Can you work these out from the model? Positions are in its coordinate system, mm. Coordinates: 2 decimals unless noted, no trailing zeros. Order: outer loops, then holes, each group sorted by start corner. A loop starts at its lowest first (then second) coordinate and runs counter-clockwise, first axis right, second up.
```python
from build123d import *

# Parameters (mm, degrees)
SKETCH_1_W                  = 85
SKETCH_1_H                  = 90
EXTRUDE_1_DEPTH             = 80
SKETCH_2_W                  = 75
SKETCH_2_H                  = 80
CUT_EXTRUDE_1_DEPTH         = 148.39402973
HOLE_WIZARD_6_6_6_6_1_D     = 6.6
HOLE_WIZARD_6_0_6_1_D       = 6
HOLE_WIZARD_6_0_6_1_DEPTH   = 85
HOLE_WIZARD_2_0_2_1_D       = 2
HOLE_WIZARD_4_5_4_5_1_D     = 4.5
HOLE_WIZARD_4_5_4_5_1_DEPTH = 90
HOLE_WIZARD_3_4_3_4_1_D     = 3.4
HOLE_WIZARD_3_4_3_4_1_DEPTH = 90
CHAMFER_1_SIZE              = 3
CHAMFER_2_SIZE              = 2.45
CHAMFER_3_SIZE              = 1.45


with BuildPart() as part:
    # 草圖1 → 填料-伸長1 (new body)
    with BuildSketch(Plane.XZ):
        with Locations((42.5, 45)):
            Rectangle(SKETCH_1_W, SKETCH_1_H)
    extrude(amount=-EXTRUDE_1_DEPTH)

    # 草圖2 → 除料-伸長1 (cut, through all)
    with BuildSketch(Plane(origin=(0, 80, 0), x_dir=(-1, 0, 0), z_dir=(0, 1, 0))):
        with Locations((-47.5, 40)):
            Rectangle(SKETCH_2_W, SKETCH_2_H)
    extrude(amount=-CUT_EXTRUDE_1_DEPTH, mode=Mode.SUBTRACT)

    # Ø6.6 (6.6) 直徑孔1 (through all)
    with Locations(Plane(origin=(10, 0, 0), x_dir=(0, 0, -1), z_dir=(1, 0, 0))):
        with Locations((-38.807552288, 10.023708227), (-60.353251324, 17.960372949), (-69.976291773, 38.807552288), (-62.039627051, 60.353251324), (-41.192447712, 69.976291773), (-19.646748676, 62.039627051), (-10.023708227, 41.192447712), (-17.960372949, 19.646748676)):
            Hole(HOLE_WIZARD_6_6_6_6_1_D / 2)

    # Ø6.0 (6) 直徑孔1
    with Locations(Plane.ZY):
        with Locations((12.761847554, 52.57310826), (67.238152446, 27.42689174)):
            Hole(HOLE_WIZARD_6_0_6_1_D / 2, depth=HOLE_WIZARD_6_0_6_1_DEPTH)

    # Ø2.0 (2) 直徑孔1 (through all)
    with Locations(Plane(origin=(0, 0, 80), x_dir=(-1, 0, 0), z_dir=(0, 0, -1))):
        with Locations((-46.377364171, 55.211997886), (-65.622635829, 24.788002114)):
            Hole(HOLE_WIZARD_2_0_2_1_D / 2)

    # Ø4.5 (4.5) 直徑孔1
    with Locations(Plane.XY.offset(90)):
        with Locations((71.275302439, 31.985785415), (41.421835359, 30.77830733), (55.302862202, 57.235907255)):
            Hole(HOLE_WIZARD_4_5_4_5_1_D / 2, depth=HOLE_WIZARD_4_5_4_5_1_DEPTH)

    # Ø3.4 (3.4) 直徑孔1
    with Locations(Plane.XY.offset(90)):
        with Locations((48.134653009, 24.375137866), (38.51201718, 39.587135752)):
            Hole(HOLE_WIZARD_3_4_3_4_1_D / 2, depth=HOLE_WIZARD_3_4_3_4_1_DEPTH)

    # 導角1
    chamfer_1_edges = [part.edges().sort_by_distance(p)[0] for p in [
        (10, 19.646748676, 14.660372949),
        (10, 41.192447712, 6.723708227),
        (10, 62.039627051, 16.346748676),
        (10, 69.976291773, 37.892447712),
        (10, 60.353251324, 58.739627051),
        (10, 38.807552288, 66.676291773),
        (10, 17.960372949, 57.053251324),
        (10, 10.023708227, 35.507552288),
    ]]
    chamfer(chamfer_1_edges, length=CHAMFER_1_SIZE)

    # 導角2
    chamfer_2_edges = [part.edges().sort_by_distance(p)[0] for p in [
        (43.671835359, 30.77830733, 90),
        (73.525302439, 31.985785415, 90),
        (57.552862202, 57.235907255, 90),
    ]]
    chamfer(chamfer_2_edges, length=CHAMFER_2_SIZE)

    # 導角3
    chamfer_3_edges = [part.edges().sort_by_distance(p)[0] for p in [
        (40.21201718, 39.587135752, 90),
        (49.834653009, 24.375137866, 90),
    ]]
    chamfer(chamfer_3_edges, length=CHAMFER_3_SIZE)


solid = part.part
```
1. Imagine slicing it at A-A on z = 52.5. Please give me the cut outline in (x, y), then the cut area to 3 significant figures.
Completed:
outline: (0, 0) - (10, 0) - (10, 80) - (0, 80) - close
area: 800 mm2
2. I'm going to push flat-ended pins straight in: pin 1 (2.5 mm diameter, centred on x = 65.62, y = 24.79, fed in from -Z); pin 2 (5 mm diameter, centred on y = 29, z = 58.5, fed in from +X); pin 3 (4.5 mm diameter, centred on x = 38.51, y = 39.59, fed in from +Z). Where does each tip first touch, or does it pass through?
Completed:
pin 1: stops at z = 80
pin 2: stops at x = 10
pin 3: stops at z = 89.1
3. Imagine slicing it at C-C on x = 14. Please give me the cut outline in (y, z).
Completed:
outline: (0, 80) - (80, 80) - (80, 90) - (0, 90) - close
4. Imagine slicing it at B-B on z = 19.5. Give the number of separate pieces and of enclosed holes in the cut face, then the cut area to 3 significant figures.
Completed:
separate pieces: 3
enclosed holes: 0
area: 657 mm2
5. Please list where these lines run through material, in increasing order: probe 1 along Y at (x, z) = (4.5, 61.5); probe 2 along Z at (x, y) = (17, 61); probe 3 along X at (y, z) = (51.5, 35).
Completed:
probe 1: y = 0 to 14.87, 21.05 to 57.1, 63.61 to 80
probe 2: z = 80 to 90
probe 3: x = 0 to 10
6. Thinking about a two-plate mould opening in Z: for faces 1 (the conical face through (7.19, 10.18, 35.32)), 2 (the cylindrical face through (49.484, 23.341, 84.215)), 3 (the flat face through (5, 39, 0)), which applies, pulls with the +Z half, pulls with the -Z half, needs draft (parallel to the pull), parting line crosses it, or undercut?
Completed:
face 1: undercut
face 2: needs draft
face 3: pulls with the -Z half
